Here's how the part is built. I have some questions about the finished solid (model axes, mm). A direction names the side the tool comes from. Coordinates: 2 decimals unless noted, no trailing zeros. Order: outer loops, then holes, each group sorted by start corner. A loop starts at its lowest first (then second) coordinate and runs counter-clockwise, first axis right, second up. Notation, with made-up numbers: M 31.5,64.25 L 84.5,64.25 A30 ccw 84.5,94.25 Z; hole C -32.5,78 d1. An arc over 180 degrees is marked long. Answer as CSV lines item,"result". Start each with the question number.
Autodesk Inventor part; units mm, degrees
ref_plane "YZ Plane" through (0, 0, 0) normal (1, 0, 0) x (0, 1, 0)
ref_plane "XZ Plane" through (0, 0, 0) normal (0, 1, 0) x (-1, 0, 0)
ref_plane "XY Plane" through (0, 0, 0) normal (0, 0, 1) x (1, 0, 0)
sketch "Sketch1" plane through (0, 0, 0) normal (0, 1, 0) x (-1, 0, 0)
  line L0 (0, 0) -> (-205.994, 0)
  line L1 (-205.994, 0) -> (-205.994, -228.854)
  line L2 (-205.994, -228.854) -> (0, -228.854)
  line L3 (0, -228.854) -> (0, 0)
  line L4 (-209.169, -232.029) -> (3.175, -232.029)
  line L5 (3.175, -232.029) -> (3.175, 3.175)
  line L6 (3.175, 3.175) -> (-209.169, 3.175)
  line L7 (-209.169, 3.175) -> (-209.169, -232.029)
  dimension "d0" = 205.994
  dimension "d1" = 228.854
  dimension "d2" = 3.175
  dimension "d3" = 3.175
  dimension "d4" = 3.175
  dimension "d5" = 3.175
extrude "Extrusion2" add sketch "Sketch1" along normal blind 25.4
sketch "Sketch2" plane through (0, 25.4, 0) normal (0, 1, 0) x (1, 0, 0)
  line L0 (-3.175, 232.029) -> (-3.175, -3.175)
  line L1 (-3.175, -3.175) -> (209.169, -3.175)
  line L2 (209.169, -3.175) -> (209.169, 232.029)
  line L3 (209.169, 232.029) -> (-3.175, 232.029)
  point P0 (0, 0)
extrude "Extrusion3" add sketch "Sketch2" along normal blind 3.175
sketch "Sketch4" plane through (0, 25.4, 0) normal (0, -1, 0) x (1, 0, 0)
  point P0 (0, 0)
properties part number "FishTankLid"
1) I need wall thicknesses on line 1 (X direction, y = 18.75, z = -21) (3 decimals); line 2 (Z direction, x = 188.5, y = 9.5) (3 decimals); line 3 (Y direction, x = 69.5, z = -212) (3 decimals). Which ranges of each line are inside material? Lowest first, please. Write a range as [from, to].
2) Which directions (+Z, -Z, +X, -X, +Y, -Y) give clear straight access to the entire face, cutting with the end or side of a thin tool? Please do faces 1 (the face through (0, 13, -116)), 2 (the face through (102, 14, 3.175)).
3) Suppose I cut it at C-C on z = -211. Please give me the cut outline in (x, y) (3 decimals), plus the area to 3 significant figures.
4) Suppose I cut it at B-B on x = 151. Please give me the cut outline in (y, z) (3 decimals), plus the area to 3 significant figures.
5) If we mould it in two halves opening along Z, with no side actions, what happens to faces 3 (the face through (104, 14, -232.029)), 4 (the face through (104, 13, -228.854)), 5 (the face through (-3.175, 14, -116))? For each: released by +Z, released by -Z, zero draft, split by the parting line, or undercut.
6) Suppose I cut it at A-A on y = 20. Please give me the cut outline in (x, z) (3 decimals), plus the area to 3 significant figures.
Output:
1,line 1,"[-3.175, 0], [205.994, 209.169]"
1,line 2,"[-232.029, -228.854], [0, 3.175]"
1,line 3,"[25.4, 28.575]"
2,face 1,"-Y"
2,face 2,"+Z, +X, -X, +Y, -Y"
3,outline,"M -3.175,0 L 0,0 L 0,25.4 L 205.994,25.4 L 205.994,0 L 209.169,0 L 209.169,28.575 L -3.175,28.575 Z"
3,area,"835 mm²"
4,outline,"M 0,-232.029 L 28.575,-232.029 L 28.575,3.175 L 0,3.175 L 0,0 L 25.4,0 L 25.4,-228.854 L 0,-228.854 Z"
4,area,"908 mm²"
5,face 3,"released by -Z"
5,face 4,"undercut"
5,face 5,"zero draft"
6,outline,"M -3.175,-232.029 L 209.169,-232.029 L 209.169,3.175 L -3.175,3.175 Z; hole M 0,-228.854 L 205.994,-228.854 L 205.994,0 L 0,0 Z"
6,area,"2,800 mm²"
